Source: CAD feature listing. Evaluate the final solid. Frame: model axes, mm. A direction names the side the tool comes from. Give positions to 0.01 mm unless a question says otherwise; leave off trailing zeros. Write each loop counter-clockwise with the first axis right and the second up, starting at its lowest first coordinate (ties: lowest second). Pieces come first, ordered by that corner, then holes.
```python
from build123d import *

# Parameters (mm, degrees)
F1_DEPTH = 3.12
F2_R     = 2.44
F3_DEPTH = 1.5
F5_DEPTH = 4.68
F6_R     = 3.235
F6_R_2   = 2.45
F7_DEPTH = 4.5
F9_DEPTH = 5


# Not quite as in the source:
# - the program builds the solid bodies; features that only make, move or delete a surface that nothing else refers to are left out


with BuildPart() as f1:
    # F0 (on Front) → F1 (new body)
    with BuildSketch(Plane.XZ):
        Polygon((14.9867535406, 12.4322535499), (-0.8932464594, 12.4322535499), (-0.8932464594, 5.6322535499), (-0.8932464594, 5.0706164911), (-3.7561513018, 5.0706164911), (-3.7561513018, 2.860605251), (-0.8932464594, 2.860605251), (-0.8932464594, -3.4477464501), (14.9867535406, -3.4477464501), (14.9867535406, 2.860605251), (18.5687988997, 2.860605251), (18.5687988997, 5.0706164911), (14.9867535406, 5.0706164911), (14.9867535406, 5.5522535499), align=None)
    extrude(amount=F1_DEPTH)

    # F2 (on Front) → F3 (join)
    with BuildSketch(Plane.XZ):
        with Locations((11.2367535406, 8.6822535499)):
            Circle(F2_R)
        with Locations((3.1867535406, 8.6822535499)):
            Circle(F2_R)
        with Locations((3.1867535406, 0.6322535499)):
            Circle(F2_R)
        with Locations((11.2367535406, 0.6322535499)):
            Circle(F2_R)
    extrude(amount=-F3_DEPTH)

    # F4 (on Front) → F5 (join)
    with BuildSketch(Plane.XZ):
        Polygon((0.5067535406, 5.13), (0.5067535406, 11.0322535499), (13.5867535406, 11.0322535499), (13.5867535406, 5.13), (14.9343172088, 5.13), (14.9343172088, 8.03), (14.9343172088, 12.5052658841), (-0.8757988689, 12.5052658841), (-1.0476475582, 8.03), (-4.6052209849, 5.9285708389), (-4.6052209849, 1.8285708389), (-1.0476475582, 0), (-0.8757988689, -3.3894693479), (14.9343172088, -3.3894693479), (14.9343172088, 0), (14.9343172088, 2.9), (13.5867535406, 2.9), (13.5867535406, -2.0477464501), (0.5067535406, -2.0477464501), (0.5067535406, 2.9), (-2.4232464594, 2.9), (-2.4232464594, 5.13), align=None)
        Polygon((14.9343172088, 8.03), (14.9343172088, 5.13), (16.5167535406, 5.13), (16.5167535406, 2.9), (14.9343172088, 2.9), (14.9343172088, 0), (18.4918906356, 1.8285708389), (18.4918906356, 5.9285708389), align=None)
    extrude(amount=F5_DEPTH)

    # F6 (on Front) → F7 (join)
    with BuildSketch(Plane.XZ):
        with Locations((7.094095153, 4.4974250309)):
            Circle(F6_R)
        with Locations((7.094095153, 4.4974250309)):
            Circle(F6_R_2, mode=Mode.SUBTRACT)
    extrude(amount=F7_DEPTH)

    # F8 (on face) → F9 (join)
    with BuildSketch(Plane.YZ.offset(18.5687988997)):
        with BuildLine():
            ThreePointArc((-0.7456844895, 3.608182552), (-0.8395787407, 4.1214828522), (-1.1091013145, 4.5683059836))
            Line((-1.1091013145, 4.5683059836), (-3.2822676645, 2.6480591205))
            ThreePointArc((-3.2822676645, 2.6480591205), (-1.6823841893, 2.2520768032), (-0.7456844895, 3.608182552))
        make_face()
        with BuildLine():
            Line((-3.2822676645, 2.6480591205), (-1.1091013145, 4.5683059836))
            ThreePointArc((-1.1091013145, 4.5683059836), (-3.1558079211, 4.694765727), (-3.2822676645, 2.6480591205))
        make_face()
    extrude(amount=F9_DEPTH)


solid = f1.part
```
1. Section query C-C (y = -2.5). Give the number of separate pieces and of enclosed holes in the cut face, plus the area to 3 significant figures.
2. Pin query (flat end, axial travel): P1, Ø2, axis at y = -2.5, z = 9.5, coming from the +X side; P2, Ø1, axis at x = 19.5, z = 2, coming from the +Y side; P3, Ø3, axis at y = 0.5, z = 4, coming from the -X side; P4, Ø4, axis at x = 10.5, z = 4.5, coming from the -Y side. Return the tip coordinate at first contact, or that it passes through.
3. Section query D-D (x = 13.25). Return loops of the section in (y, z).
4. Section query B-B (z = -1.5). Return loops of the section in (x, y), plus the area to 3 significant figures.
5. Access query for faces 1 (the flat face through (7, 0, 5)), 2 (the flat face through (14.987, -2, 10)), 3 (the flat face through (0.507, -4, 0)). Directions: +Z, -Z, +X, -X, +Y, -Y. A direction counts if a zero-diameter tool reaches every point of the face in a straight line with its end or side. Return the directions, or none.
6. Line query: probe 1 along Z at (x, y) = (1.75, -4.5); probe 2 along X at (y, z) = (-4.25, 2.5); probe 3 along Y at (x, z) = (12, 10.5). Output: solid intervals per line, ascending.
7. Section query A-A (x = -0.5). Return loops of the section in (y, z), plus the area to 3 significant figures.
The answers:
1. separate pieces: 1
1. enclosed holes: 2
1. area: 312 mm2
2. P1: stops at x = 14.99
2. P2: stops at y = -1.26
2. P3: stops at x = -4.61
2. P4: stops at y = -4.5
3. outline: (-4.68, -3.39) - (-3.12, -3.39) - (-3.12, -3.45) - (0, -3.45) - (0, -0.75) - (1.5, -0.75) - (1.5, 2.01) - (0, 2.01) - (0, 7.3) - (1.5, 7.3) - (1.5, 10.06) - (0, 10.06) - (0, 12.51) - (-4.68, 12.51) - (-4.68, 11.03) - (-3.12, 11.03) - (-3.12, -2.05) - (-4.68, -2.05) - close
4. outline: (-0.97, -4.68) - (0.51, -4.68) - (0.51, -3.12) - (13.59, -3.12) - (13.59, -4.68) - (14.93, -4.68) - (14.93, -3.12) - (14.99, -3.12) - (14.99, 0) - (12.42, 0) - (12.42, 1.5) - (10.05, 1.5) - (10.05, 0) - (4.37, 0) - (4.37, 1.5) - (2, 1.5) - (2, 0) - (-0.97, 0) - close
4. area: 61.3 mm2
5. face 1: +Y
5. face 2: +Z, +X, +Y, -Y
5. face 3: -Y
6. probe 1: z = -3.39 to -2.05, 11.03 to 12.51
6. probe 2: x = -4.61 to 0.51, 4.55 to 5.68, 8.51 to 9.64, 13.59 to 18.49
6. probe 3: y = -3.12 to 1.5
7. outline: (-4.68, -3.39) - (-3.12, -3.39) - (-3.12, -3.45) - (0, -3.45) - (0, 12.51) - (-4.68, 12.51) - (-4.68, 5.13) - (-3.12, 5.13) - (-3.12, 2.9) - (-4.68, 2.9) - close
7. area: 71.1 mm2
